Model file for the job. Use its own axes, mm. A direction names the side the tool comes from. Give positions to 0.01 mm unless a question says otherwise; leave off trailing zeros. Loops run counter-clockwise (first coordinate to the right, second up) from the corner with the lowest first, then second, coordinate; pieces in that order, holes last. Notation, with made-up numbers: M 55,-11.75 L 66,-11.75 A18 cw 66,-3.75 Z; hole C 89.5,67.5 d2. An arc over 180 degrees is marked long. Answer in a Markdown table with one row per item.
```python
from build123d import *

# Parameters (mm, degrees)
BOSS_EXTRUDE1_DEPTH       = 10
FILLET1_R                 = 40
M4X0_7_TAPPED_HOLE1_D     = 3.3
M4X0_7_TAPPED_HOLE1_DEPTH = 17.839823294
M3_CLEARANCE_HOLE3_D      = 3.4
M3_CLEARANCE_HOLE3_DEPTH  = 10
SKETCH23_R                = 11.5
CUT_EXTRUDE3_DEPTH        = 5
CIRPATTERN2_COUNT         = 3
FILLET2_R                 = 1.5


with BuildPart() as part:
    # Sketch1 → Boss-Extrude1 (new body)
    with BuildSketch(Plane.XY):
        Polygon((7, 36), (-7, 36), (-7, 4.041451884), (-34.676914536, -11.937822174), (-27.676914536, -24.062177826), (0, -8.082903769), (27.676914536, -24.062177826), (34.676914536, -11.937822174), (7, 4.041451884), align=None)
    extrude(amount=BOSS_EXTRUDE1_DEPTH)

    # Fillet1
    fillet1_edges = [part.edges().sort_by_distance(p)[0] for p in [
        (7, 4.041451884, 5),
        (0, -8.082903769, 5),
        (-7, 4.041451884, 5),
    ]]
    fillet(fillet1_edges, radius=FILLET1_R)

    # M4x0.7 Tapped Hole1
    with Locations(Plane.ZY.offset(7)):
        with Locations((5, 31.567731326)):
            m4x0_7_tapped_hole1 = Hole(M4X0_7_TAPPED_HOLE1_D / 2, depth=M4X0_7_TAPPED_HOLE1_DEPTH)

    # M3 Clearance Hole3
    with Locations(Plane.XY.offset(10)):
        with Locations((0, 0), (0, 8), (5.656854249, 5.656854249), (8, 0), (5.656854249, -5.656854249), (0, -8), (-5.656854249, -5.656854249), (-8, 0), (-5.656854249, 5.656854249)):
            Hole(M3_CLEARANCE_HOLE3_D / 2, depth=M3_CLEARANCE_HOLE3_DEPTH)

    # Sketch23 → Cut-Extrude3 (cut)
    with BuildSketch(Plane.XY.offset(10)):
        Circle(SKETCH23_R)
    extrude(amount=-CUT_EXTRUDE3_DEPTH, mode=Mode.SUBTRACT)

    # CirPattern2: M4x0.7 Tapped Hole1 ×3 about axis
    cirpattern2_axis = Axis((0, 0, 5), (0, 0, 1))
    for i in range(1, CIRPATTERN2_COUNT):
        add(m4x0_7_tapped_hole1.rotate(cirpattern2_axis, i * 360 / CIRPATTERN2_COUNT), mode=Mode.SUBTRACT)

    # Fillet2
    fillet2_edges = [part.edges().sort_by_distance(p)[0] for p in [
        (30.838457268, -9.721687836, 0),
        (31.176914536, -18, 0),
        (-23.838457268, -21.846043489, 0),
        (-31.176914536, -18, 0),
        (-7, 31.567731326, 0),
        (-31.176914536, -18, 10),
        (-7, 36, 5),
        (7, 36, 5),
        (34.676914536, -11.937822174, 5),
        (27.676914536, -24.062177826, 5),
        (-27.676914536, -24.062177826, 5),
        (-34.676914536, -11.937822174, 5),
        (-23.838457268, -21.846043489, 10),
        (31.176914536, -18, 10),
        (23.838457268, -21.846043489, 0),
        (23.838457268, -21.846043489, 10),
        (30.838457268, -9.721687836, 10),
        (7, 31.567731326, 0),
        (7, 31.567731326, 10),
        (-30.838457268, -9.721687836, 0),
        (-30.838457268, -9.721687836, 10),
        (0, -14.270925304, 0),
        (0, -14.270925304, 10),
        (12.358983849, 7.135462652, 0),
        (12.358983849, 7.135462652, 10),
        (-12.358983849, 7.135462652, 0),
        (-12.358983849, 7.135462652, 10),
        (0, 36, 10),
        (-7, 31.567731326, 10),
        (0, 36, 0),
    ]]
    fillet(fillet2_edges, radius=FILLET2_R)


solid = part.part
```
Q1. Mould opens along X. For faces 1 (the face through (29.92, -9.71, 0.43)), 2 (the face through (-23.37, -21.055, 0.428)), 3 (the face through (-0.08, 35.57, 9.55)), 4 (the face through (-30.01, -9.76, 9.57)) say: released by +X, released by -X, zero draft, split by the parting line, or undercut.
Reported:
| item | result |
|---|---|
| face 1 | released by +X |
| face 2 | undercut |
| face 3 | zero draft |
| face 4 | released by -X |
Q2. Saw through at A-A (z = 9.25). Give the cut face in (x, y).
Reported:
| item | result |
|---|---|
| outline | M -33.75,-13.14 L -28.25,-22.66 A1.3 ccw -26.48,-23.14 L -20.1,-19.46 A40.2 cw 20.1,-19.46 L 26.48,-23.14 A1.3 ccw 28.25,-22.66 L 33.75,-13.14 A1.3 ccw 33.28,-11.36 L 26.9,-7.68 A40.2 cw 6.8,27.14 L 6.8,34.5 A1.3 ccw 5.5,35.8 L -5.5,35.8 A1.3 ccw -6.8,34.5 L -6.8,27.14 A40.2 cw -26.9,-7.68 L -33.28,-11.36 A1.3 ccw Z; hole C 0,0 d23 |
Q3. Drop flat-ended pins along their axis: pin 1 (6 mm diameter, centred on x = 22, y = -11, fed in from -Z); pin 2 (1 mm diameter, centred on x = 23.5, z = 1.5, fed in from -Y); pin 3 (20.5 mm diameter, centred on x = 0, y = 0, fed in from +Z); pin 4 (2 mm diameter, centred on y = 6, z = 7, fed in from +X). Give the stop position or say it passes through.
Reported:
| item | result |
|---|---|
| pin 1 | z = 0 |
| pin 2 | y = -21.94 |
| pin 3 | z = 5 |
| pin 4 | x = 13.68 |
Q4. Saw through at B-B (y = -16). Give the number of separate pieces and of enclosed holes in the cut face, and give its area (3 significant figures).
Reported:
| item | result |
|---|---|
| separate pieces | 2 |
| enclosed holes | 2 |
| area | 386 mm² |
Q5. Probe probe 1 along Y at (x, z) = (0, 1.3); probe 2 along Y at (x, z) = (0, 7.25); probe 3 along Y at (x, z) = (0, 6.45). List the from-to ranges inside material, lowest first.
Reported:
| item | result |
|---|---|
| probe 1 | -14.26 to -9.7, -6.3 to -1.7, 1.7 to 6.3, 9.7 to 35.99 |
| probe 2 | -14.27 to -11.5, 11.5 to 36 |
| probe 3 | -14.27 to -11.5, 11.5 to 30.78, 32.36 to 36 |
Q6. 3-axis set-ups, long thin cutter, end or side, ignore diameter. For faces 5 (the face through (-23.37, -21.055, 9.572)), 6 (the face through (-6.55, 30.77, 9.57)), 7 (the face through (34.07, -12.08, 5.05)), 8 (the face through (22.44, -21.04, 4.17)), 9 (the face through (7, 30, 6)): which of +Z, -Z, +X, -X, +Y, -Y reach the whole face in a straight line?
Reported:
| item | result |
|---|---|
| face 5 | +Z, -Y |
| face 6 | +Z, -X, +Y |
| face 7 | +Z, -Z, +X |
| face 8 | +Z, -Z, -Y |
| face 9 | +Z, -Z, +X, +Y |
